Geometry: final body of the model. Coordinates: model frame, mm. A direction names the side the tool comes from. Coordinates: 2 decimals unless noted, no trailing zeros. Loops run counter-clockwise (first coordinate to the right, second up) from the corner with the lowest first, then second, coordinate; pieces in that order, holes last. Notation, with made-up numbers: (49.25, -7) - (92.25, -7) arc R25 ccw to (92.25, 16) - close; hole circle Ø6 at (14, 81). An arc over 180 degrees is marked (long way). Write each question's results on one line, items separated by ' | '. Start each with the question number.
from build123d import *

# Parameters (mm, degrees)
BOSS_EXTRUDE1_DEPTH = 5
SKETCH2_R           = 1.15
CUT_EXTRUDE1_DEPTH  = 87.690729745
FILLET1_R           = 5
FILLET3_R           = 1
FILLET12_R          = 5
FILLET14_R          = 1
FILLET15_R          = 10
FILLET16_R          = 10
BOSS_EXTRUDE2_DEPTH = 5
FILLET17_R          = 0.2
FILLET18_R          = 15


with BuildPart() as part:
    # Sketch1 → Boss-Extrude1 (new body)
    with BuildSketch(Plane.XY):
        with BuildLine():
            Line((-6.5, 17.5), (-6.5, 11.5))
            Line((-6.5, 11.5), (6.5, 11.5))
            Line((6.5, 11.5), (6.5, -11.5))
            Line((6.5, -11.5), (-6.5, -11.5))
            Line((-6.5, -11.5), (-6.5, -17.5))
            Line((-6.5, -17.5), (9.5, -17.5))
            ThreePointArc((9.5, -17.5), (15.62941886, -44.673850811), (14.328125353, -72.5))
            Line((14.328125353, -72.5), (14.328125353, -82.5))
            Line((14.328125353, -82.5), (18.328125353, -82.5))
            Line((18.328125353, -82.5), (18.328125353, -72.5))
            ThreePointArc((18.328125353, -72.5), (25.796688212, -26.509948672), (10.5, 17.5))
            Line((10.5, 17.5), (-6.5, 17.5))
        make_face()
    extrude(amount=BOSS_EXTRUDE1_DEPTH)

    # Sketch2 → Cut-Extrude1 (cut, through all)
    with BuildSketch(Plane.XY.offset(5)):
        with Locations((0.25, 13.9)):
            Circle(SKETCH2_R)
        with Locations((0.25, -13.9)):
            Circle(SKETCH2_R)
    extrude(amount=-CUT_EXTRUDE1_DEPTH, mode=Mode.SUBTRACT)

    # Fillet1
    fillet1_edges = [part.edges().sort_by_distance(p)[0] for p in [
        (10.5, 17.5, 2.5),
    ]]
    fillet(fillet1_edges, radius=FILLET1_R)

    # Fillet3
    fillet3_edges = [part.edges().sort_by_distance(p)[0] for p in [
        (-6.5, -17.5, 2.5),
        (-6.5, -11.5, 2.5),
        (-6.5, 11.5, 2.5),
        (-6.5, 17.5, 2.5),
    ]]
    fillet(fillet3_edges, radius=FILLET3_R)

    # Fillet12
    fillet12_edges = [part.edges().sort_by_distance(p)[0] for p in [
        (18.328125353, -72.5, 2.5),
    ]]
    fillet(fillet12_edges, radius=FILLET12_R)

    # Fillet14
    fillet14_edges = [part.edges().sort_by_distance(p)[0] for p in [
        (18.328125353, -82.5, 2.5),
        (14.328125353, -82.5, 2.5),
    ]]
    fillet(fillet14_edges, radius=FILLET14_R)

    # Fillet15
    fillet15_edges = [part.edges().sort_by_distance(p)[0] for p in [
        (14.328125353, -72.5, 2.5),
    ]]
    fillet(fillet15_edges, radius=FILLET15_R)

    # Fillet16
    fillet16_edges = [part.edges().sort_by_distance(p)[0] for p in [
        (9.5, -17.5, 2.5),
    ]]
    fillet(fillet16_edges, radius=FILLET16_R)

    # Sketch3 → Boss-Extrude2 (add)
    with BuildSketch(Plane.XY.offset(5)):
        with BuildLine():
            Line((-5.5, 17.5), (7.758219973, 17.5))
            Line((7.758219973, 17.5), (7.758219973, 24.5))
            ThreePointArc((7.758219973, 24.5), (1.666211007, 19.982713789), (-5.5, 17.5))
        make_face()
    extrude(amount=-BOSS_EXTRUDE2_DEPTH)

    # Fillet17
    fillet17_edges = [part.edges().sort_by_distance(p)[0] for p in [
        (7.758219973, 24.5, 2.5),
    ]]
    fillet(fillet17_edges, radius=FILLET17_R)

    # Fillet18
    fillet18_edges = [part.edges().sort_by_distance(p)[0] for p in [
        (7.758219973, 17.5, 2.5),
    ]]
    fillet(fillet18_edges, radius=FILLET18_R)


solid = part.part
1) Section query B-B on x = 5. Output: boundary loops of the cut face in (y, z).
2) Material intervals for line 1 (Y direction, x = 0.25, z = 3.3); line 2 (Y direction, x = 1, z = 2.3); line 3 (Y direction, x = 2, z = 2), sorted ascending. Write a range as [from, to].
3) Section query A-A on y = 13.9. Output: boundary loops of the cut face in (x, z).
4) Section query C-C on x = 0.25. Output: boundary loops of the cut face in (y, z), and give its area (3 significant figures).
5) Pin query (flat end, axial travel): pin 1 Ø2.5 at (x, y) = (0.25, -13.9) entering from -Z; pin 2 Ø1 at (y, z) = (-54.5, 4) entering from +X; pin 3 Ø3 at (x, z) = (8, 2.5) entering from -Y. Return the tip coordinate at first contact, or that it passes through.
6) Section query D-D on z = 2.35. Count the separate pieces of the cut face and the enclosed holes in it, and give its area (3 significant figures).
7) Access query for faces 5 (the cylindrical face through (14.364, -72.535, 2.535)), 6 (the cylindrical face through (18.43, -72.52, 2.54)), 7 (the flat face through (14.328, -77, 2)). Directions: +Z, -Z, +X, -X, +Y, -Y. A direction counts if a zero-diameter tool reaches every point of the face in a straight line with its end or side. Return the directions, or none.
8) Pull-direction query (Y, two-part tool) for faces 1 (the cylindrical face through (15.85, -47.71, 2.46)), 2 (the cylindrical face through (25.92, -28.05, 2.46)), 3 (the flat face through (16, -82.5, 2)), 4 (the flat face through (18.328, -78, 2)); classes: released by +Y, released by -Y, zero draft, split by the parting line, or undercut.
Returned:
1) outline: (-17.88, 0) - (-11.5, 0) - (-11.5, 5) - (-17.88, 5) - close; (11.5, 0) - (22.1, 0) - (22.1, 5) - (11.5, 5) - close
2) line 1: y = [-17.5, -15.05], [-12.75, -11.5], [11.5, 12.75], [15.05, 19.29] | line 2: y = [-17.5, -14.77], [-13.03, -11.5], [11.5, 13.03], [14.77, 19.64] | line 3: y = [-17.5, -11.5], [11.5, 20.16]
3) outline: (-6.5, 0) - (-0.9, 0) - (-0.9, 5) - (-6.5, 5) - close; (1.4, 0) - (12.76, 0) - (12.76, 5) - (1.4, 5) - close
4) outline: (-17.5, 0) - (-15.05, 0) - (-15.05, 5) - (-17.5, 5) - close; (-12.75, 0) - (-11.5, 0) - (-11.5, 5) - (-12.75, 5) - close; (11.5, 0) - (12.75, 0) - (12.75, 5) - (11.5, 5) - close; (15.05, 0) - (19.29, 0) - (19.29, 5) - (15.05, 5) - close | area: 46.0 mm²
5) pin 1: stops at z = 0 | pin 2: stops at x = 24.18 | pin 3: stops at y = -20.58
6) separate pieces: 1 | enclosed holes: 2 | area: 1,210 mm²
7) face 5: +Z, -Z, -X | face 6: +Z, -Z, +X, -Y | face 7: +Z, -Z, -X, -Y
8) face 1: undercut | face 2: split by the parting line | face 3: released by -Y | face 4: zero draft
